from build123d import *

# Parameters (mm, degrees)
AUFSATZ_LINEAR_AUSTRAGEN1_DEPTH = 10
SKIZZE2_R                       = 5
SCHNITT_LINEAR_AUSTRAGEN1_DEPTH = 2


with BuildPart() as part:
    # Skizze1 → Aufsatz-Linear austragen1 (new body, symmetric)
    with BuildSketch(Plane(origin=(0, 0, 0), x_dir=(1, 0, 0), z_dir=(0, 1, 0))):
        Polygon((-5, 0), (-10.176380902, -19.318516526), (-12.108232555, -18.800878436), (-6.534653976, 2), (6.534653976, 2), (12.108232555, -18.800878436), (10.176380902, -19.318516526), (5, 0), align=None)
    extrude(amount=AUFSATZ_LINEAR_AUSTRAGEN1_DEPTH, both=True)

    # Skizze2 → Schnitt-Linear austragen1 (cut)
    with BuildSketch(Plane(origin=(6.596915162, 0, -1.76763809), x_dir=(-0.258819045, 0, -0.965925826), z_dir=(0.965925826, 0, -0.258819045))):
        with Locations((-10.526768238, 0)):
            Circle(SKIZZE2_R)
    schnitt_linear_austragen1 = extrude(amount=-SCHNITT_LINEAR_AUSTRAGEN1_DEPTH, mode=Mode.SUBTRACT)

    # Spiegeln1: Schnitt-Linear austragen1 across plane
    add(schnitt_linear_austragen1.mirror(Plane(origin=(0, 0, 0), x_dir=(0, 0, 1), z_dir=(1, 0, 0))), mode=Mode.SUBTRACT)


solid = part.part
Geometry check sheet. Reference: the model listing, model coordinates, mm. A direction names the side the tool comes from. Give positions to 0.01 mm unless a question says otherwise; leave off trailing zeros. Write each loop counter-clockwise with the first axis right and the second up, starting at its lowest first coordinate (ties: lowest second). Pieces come first, ordered by that corner, then holes. Notation, with made-up numbers: M 35.25,-10 L 56.25,-10 A22 cw 56.25,28 Z; hole C -33,28 d3. An arc over 180 degrees is marked long. Answer as CSV lines item,"result". Start each with the question number.
Q1. Material ranges on L1, parallel to X at y = 0, z = 14.25; L2, parallel to X at y = 7.5, z = 16.25; L3, parallel to Z at x = 4.75, y = 7.25, recorded low to high.
Q2. Section check C-C, the plane y = -7. Record the cut outline in (x, z).
Q3. Section check A-A, the plane y = 2.5. Record the cut outline in (x, z), then the cut area to 3 significant figures.
Q4. Section check D-D, the plane z = 7.75. Give the number of separate pieces and of enclosed holes in the cut face, then the cut area to 3 significant figures.
Q5. Release check for a two-part mould opening along Y. For faces 3 (the face through (-6.22, 10, 3.87)), 4 (the face through (8.775, 0.14, 14.087)), 5 (the face through (8.65, -4.88, 9.7)) record: pulls with the +Y half, pulls with the -Y half, needs draft (parallel to the pull), parting line crosses it, or undercut.
Q6. Tool access check on faces 1 (the face through (-8.702, -2.082, 13.817)), 2 (the face through (-11.129, 0.14, 19.063)). Record the directions out of +Z, -Z, +X, -X, +Y, -Y that give a thin tool (end or side, any length) a straight path to the whole face; none if there is none.
Q7. Section check B-B, the plane z = 16. Record the cut outline in (x, y), then the cut area to 3 significant figures.
Q8. Go/stop test with flat-tipped pins: pin 1 (1.5 mm diameter, centred on y = -7.5, z = 3.5, fed in from -X); pin 2 (8 mm diameter, centred on x = -5, z = 3, fed in from +Y); pin 3 (8 mm diameter, centred on y = -4, z = 5.5, fed in from +X). Record where each tip stops, or that it passes through.
Geometry says:
1,L1,"-10.89 to -8.82, 8.82 to 10.89"
1,L2,"-11.42 to -9.35, 9.35 to 11.42"
1,L3,"-2 to 0"
2,outline,"M -12.11,18.8 L -6.53,-2 L 6.53,-2 L 12.11,18.8 L 10.18,19.32 L 5,0 L -5,0 L -10.18,19.32 Z"
3,outline,"M -12.11,18.8 L -10.44,12.58 L -8.51,13.1 L -10.18,19.32 Z; M -8.2,4.22 L -6.53,-2 L 6.53,-2 L 8.2,4.22 L 6.27,4.74 L 5,0 L -5,0 L -6.27,4.74 Z; M 8.51,13.1 L 10.44,12.58 L 12.11,18.8 L 10.18,19.32 Z"
3,area,"71.5 mm^2"
4,separate pieces,"4"
4,enclosed holes,"0"
4,area,"42.2 mm^2"
5,face 3,"pulls with the +Y half"
5,face 4,"needs draft"
5,face 5,"undercut"
6,face 1,"+Z, +Y, -Y"
6,face 2,"+Z, -X, +Y, -Y"
7,outline,"M -11.36,-10 L -9.29,-10 L -9.29,10 L -11.36,10 Z; M 9.29,-10 L 11.36,-10 L 11.36,10 L 9.29,10 Z"
7,area,"82.8 mm^2"
8,pin 1,"x = -8.21"
8,pin 2,"y = 10"
8,pin 3,"x = 9.59"
